Check sheet for the modelled part. Datum: model origin and axes. Units: mm. Face numbers are marked on the shaded views. A direction names the side the tool comes from. Give positions to 0.01 mm unless a question says otherwise; leave off trailing zeros. Order: outer loops, then holes, each group sorted by start corner. A loop starts at its lowest first (then second) coordinate and runs counter-clockwise, first axis right, second up.
```python
from build123d import *

# Parameters (mm, degrees)
SKETCH1_W                                   = 44
SKETCH1_H                                   = 24
CROSSHEAD_BASE_DEPTH                        = 12
SHOE_UPRISER_START                          = 12
SKETCH2_W                                   = 8
SKETCH2_H                                   = 24
SHOE_UPRISER_DEPTH                          = 11
ADAPTER_BRIDGE_START                        = 12
SKETCH3_W                                   = 16
SKETCH3_H                                   = 28
ADAPTER_BRIDGE_DEPTH                        = 8
THREADED_ROD_ADAPTER_START                  = 20
SKETCH4_W                                   = 16
SKETCH4_H                                   = 16
THREADED_ROD_ADAPTER_DEPTH                  = 12
TWO_BRONZE_BUSH_HOUSINGS_DEPTH              = 48.874836814
TWO_BRONZE_BUSH_HOUSINGS_DEPTH_BACK         = 48.874836814
SKETCH5_R                                   = 5
QUARTER20_ADAPTER_MAJOR_ENVELOPE_DEPTH      = 48.874836814
QUARTER20_ADAPTER_MAJOR_ENVELOPE_DEPTH_BACK = 48.874836814
SKETCH6_R                                   = 3.175


with BuildPart() as part:
    # Sketch1 → Crosshead_Base (new body)
    with BuildSketch(Plane.XY):
        Rectangle(SKETCH1_W, SKETCH1_H)
    extrude(amount=CROSSHEAD_BASE_DEPTH)

    # Sketch2 → Shoe_Upriser (add)
    with BuildSketch(Plane.XY.offset(SHOE_UPRISER_START)):
        Rectangle(SKETCH2_W, SKETCH2_H)
    extrude(amount=SHOE_UPRISER_DEPTH)

    # Sketch3 → Adapter_Bridge (add)
    with BuildSketch(Plane.XY.offset(ADAPTER_BRIDGE_START)):
        with Locations((0, -14)):
            Rectangle(SKETCH3_W, SKETCH3_H)
    extrude(amount=ADAPTER_BRIDGE_DEPTH)

    # Sketch4 → Threaded_Rod_Adapter (add)
    with BuildSketch(Plane.XY.offset(THREADED_ROD_ADAPTER_START)):
        with Locations((0, -20)):
            Rectangle(SKETCH4_W, SKETCH4_H)
    extrude(amount=THREADED_ROD_ADAPTER_DEPTH)

    # Sketch5 → Two_Bronze_Bush_Housings (cut, two sides: drawn at the far end of the back side and taken through both)
    with BuildSketch(Plane(origin=(0, 0, 0), x_dir=(1, 0, 0), z_dir=(0, 1, 0)).offset(-TWO_BRONZE_BUSH_HOUSINGS_DEPTH_BACK)):
        with Locations(Location((-14, -6, 0), (0, 0, 270))):
            Circle(SKETCH5_R)
        with Locations(Location((14, -6, 0), (0, 0, 270))):
            Circle(SKETCH5_R)
    extrude(amount=TWO_BRONZE_BUSH_HOUSINGS_DEPTH + TWO_BRONZE_BUSH_HOUSINGS_DEPTH_BACK, mode=Mode.SUBTRACT)

    # Sketch6 → Quarter20_Adapter_Major_Envelope (cut, two sides: drawn at the far end of the back side and taken through both)
    with BuildSketch(Plane(origin=(0, 0, 0), x_dir=(1, 0, 0), z_dir=(0, 1, 0)).offset(-QUARTER20_ADAPTER_MAJOR_ENVELOPE_DEPTH_BACK)):
        with Locations(Location((0, -26, 0), (0, 0, 270))):
            Circle(SKETCH6_R)
    extrude(amount=QUARTER20_ADAPTER_MAJOR_ENVELOPE_DEPTH + QUARTER20_ADAPTER_MAJOR_ENVELOPE_DEPTH_BACK, mode=Mode.SUBTRACT)


solid = part.part
```
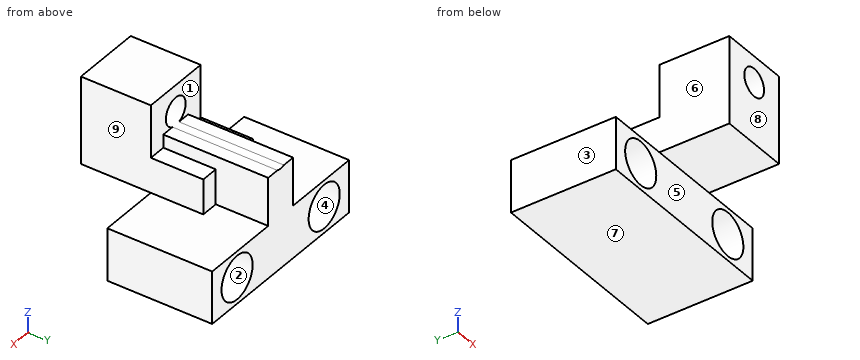
(1) Cross-section at D-D on x = -6.5. Enter the section's corners in (y, z).
Response values:
outline: (-28, 12) - (-12, 12) - (-12, 0) - (12, 0) - (12, 12) - (0, 12) - (0, 20) - (-12, 20) - (-12, 32) - (-28, 32) - close
(2) Material ranges on L1, parallel to Z at x = 14, y = 3; L2, parallel to X at y = 4, z = 6; L3, parallel to X at y = -8.5, z = 1.5, recorded low to high.
Response values:
L1: z = 0 to 1, 11 to 12
L2: x = -22 to -19, -9 to 9, 19 to 22
L3: x = -22 to -16.18, -11.82 to 11.82, 16.18 to 22
(3) Gauge pin test, flat ends, axial feed: pin 1 Ø0.9 at (x, y) = (-2.5, 4.5) entering from +Z; pin 2 Ø1.2 at (x, y) = (6, -7.5) entering from +Z; pin 3 Ø2 at (x, y) = (11.5, -1) entering from +Z. Record the tip position at first contact, or that the pin passes through.
Response values:
pin 1: stops at z = 23
pin 2: stops at z = 20
pin 3: stops at z = 12
(4) Release check for a two-part mould opening along X. For the marked faces 1, 2, 3 and 4 record: released by +X, released by -X, zero draft, split by the parting line, or undercut.
Response values:
face 1: zero draft
face 2: undercut
face 3: released by -X
face 4: undercut
(5) Cross-section at B-B on z = 26. Enter the section's corners in (x, y) (3 decimals), then the cut area to 3 significant figures.
Response values:
outline: (-8, -28) - (-3.175, -28) - (-3.175, -12) - (-8, -12) - close; (3.175, -28) - (8, -28) - (8, -12) - (3.175, -12) - close
area: 154 mm2
(6) Cross-section at C-C on y = -2. Enter the section's corners in (x, z) (3 decimals), then the cut area to 3 significant figures.
Response values:
outline: (-22, 0) - (22, 0) - (22, 12) - (8, 12) - (8, 20) - (4, 20) - (4, 23) - (1.04, 23) arc R3.175 cw to (-1.04, 23) - (-4, 23) - (-4, 20) - (-8, 20) - (-8, 12) - (-22, 12) - close; hole circle Ø10 at (-14, 6); hole circle Ø10 at (14, 6)
area: 523 mm2
(7) Cross-section at A-A on x = -14. Enter the section's corners in (y, z).
Response values:
outline: (-12, 0) - (12, 0) - (12, 1) - (-12, 1) - close; (-12, 11) - (12, 11) - (12, 12) - (-12, 12) - close
(8) Set-up check for the marked faces 5, 6, 7, 8 and 9: record each of +Z, -Z, +X, -X, +Y, -Y from which the full face is reachable in a straight line by a thin tool's end or side.
Response values:
face 5: -Z, +X, -X, -Y
face 6: +Z, -X, +Y, -Y
face 7: -Z, +X, -X, +Y, -Y
face 8: +Z, -Z, +X, -X, -Y
face 9: +Z, +X, +Y, -Y
